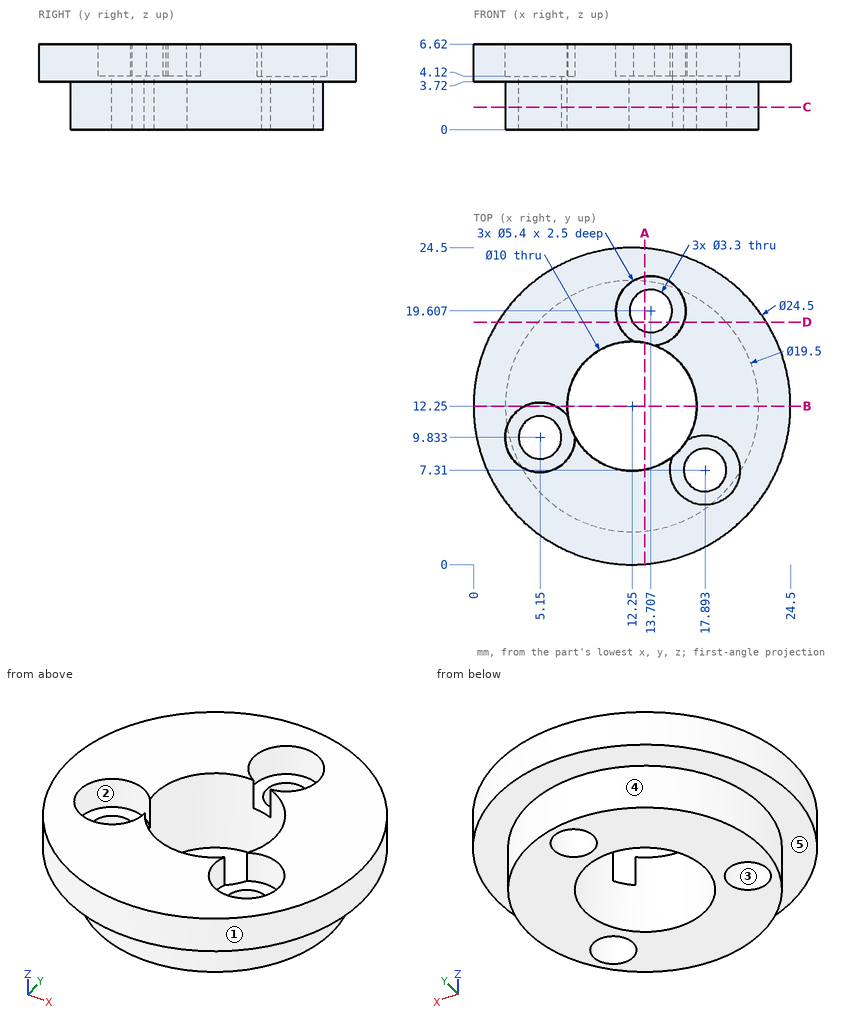
Can you work these out from the drawing? Everything is in mm from the part's minimum corner. A direction names the side the tool comes from. Round coordinates to 2 decimals unless told otherwise and drop trailing zeros. Loops run counter-clockwise (first coordinate to the right, second up) from the corner with the lowest first, then second, coordinate; pieces in that order, holes last. Notation, with made-up numbers: (43, -37) -> (93, -37) arc R15 ccw to (93, -30) -> close; hole circle Ø3 at (31, -26). An arc over 180 degrees is marked (long way). Use CSV: the item, a comma, the result in double quotes.
(1) If we mould it in two halves opening along Y, with no side actions, what happens to the marked faces 3, 4 and 5? For each: +Y half, -Y half, draft (parallel to the pull), parting line (faces both ways), or undercut.
Return value:
face 3,"undercut"
face 4,"parting line"
face 5,"draft"
(2) If I drill on probe 1 along Y at (x, z) = (13, 3.75) (1 decimal); probe 2 along X at (y, z) = (10.75, 3.25) (1 decimal); probe 3 along Y at (x, z) = (13.25, 1.5), over which ranges is the centre line in solid material (lowest first)? Write a range as [from, to].
Return value:
probe 1,"y = [0, 7.3], [17.2, 18.1], [21.1, 24.5]"
probe 2,"x = [2.6, 3.8], [6.5, 7.5], [17, 21.9]"
probe 3,"y = [2.55, 7.35], [17.15, 18.02], [21.19, 21.95]"
(3) For the marked faces 1 and 2, which set-ups out of +Z, -Z, +X, -X, +Y, -Y let a thin tool reach every point of the face, with its end or its side?
Return value:
face 1,"+Z, -Z"
face 2,"+Z"
(4) Suppose I cut it at D-D on y = 18.75. Write out the boundary of the cut face in (x, z).
Return value:
outline,"(1.87, 3.72) -> (4.98, 3.72) -> (4.98, 0) -> (12.3, 0) -> (12.3, 4.12) -> (11.15, 4.12) -> (11.15, 6.62) -> (1.87, 6.62) -> close; (15.12, 0) -> (19.52, 0) -> (19.52, 3.72) -> (22.63, 3.72) -> (22.63, 6.62) -> (16.27, 6.62) -> (16.27, 4.12) -> (15.12, 4.12) -> close"
(5) Suppose I cut it at A-A on x = 13.25. Write out the boundary of the cut face in (y, z).
Return value:
outline,"(0.04, 3.72) -> (2.55, 3.72) -> (2.55, 0) -> (7.35, 0) -> (7.35, 6.62) -> (0.04, 6.62) -> close; (17.15, 0) -> (18.02, 0) -> (18.02, 4.12) -> (17.15, 4.12) -> close; (21.19, 0) -> (21.95, 0) -> (21.95, 3.72) -> (24.46, 3.72) -> (24.46, 6.62) -> (22.27, 6.62) -> (22.27, 4.12) -> (21.19, 4.12) -> close"
(6) Will these pins go through, and if not, where does the flat tip stop? pin 1 Ø3 at (x, y) = (17.89, 7.31) entering from +Z; pin 2 Ø2 at (y, z) = (5.5, 2.5) entering from +X (1 decimal); pin 3 Ø2.5 at (x, y) = (17.5, 6.5) entering from +Z; pin 4 Ø3 at (x, z) = (3.5, 2.5) entering from -Y.
Return value:
pin 1,"passes through"
pin 2,"stops at x = 20.1"
pin 3,"stops at z = 4.12"
pin 4,"stops at y = 2.87"
(7) Suppose I cut it at B-B on y = 12.25. Write out the boundary of the cut face in (x, z).
Return value:
outline,"(0, 3.72) -> (2.5, 3.72) -> (2.5, 0) -> (7.25, 0) -> (7.25, 6.62) -> (6.35, 6.62) -> (6.35, 4.12) -> (3.95, 4.12) -> (3.95, 6.62) -> (0, 6.62) -> close; (17.25, 0) -> (22, 0) -> (22, 3.72) -> (24.5, 3.72) -> (24.5, 6.62) -> (17.25, 6.62) -> close"
(8) Suppose I cut it at C-C on z = 1.75. Write out the boundary of the cut face in (x, y).
Return value:
outline,"circle Ø19.5 at (12.25, 12.25); hole circle Ø3.3 at (5.15, 9.83); hole circle Ø10 at (12.25, 12.25); hole circle Ø3.3 at (13.71, 19.61); hole circle Ø3.3 at (17.89, 7.31)"
